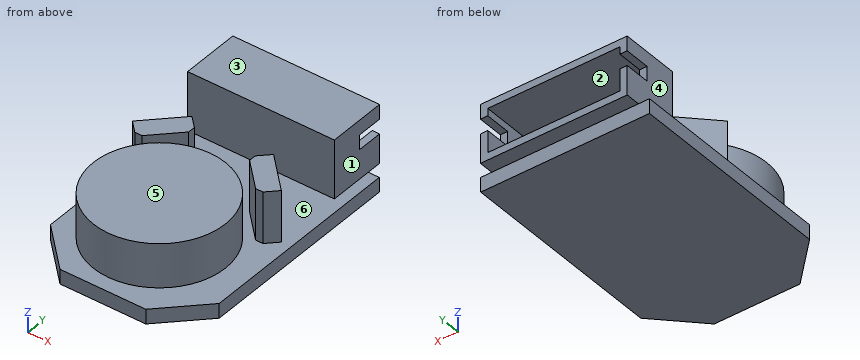
from build123d import *

# Parameters (mm, degrees)
SALIENTE_EXTRUIR1_DEPTH = 1
SALIENTE_EXTRUIR2_DEPTH = 3.5
CROQUIS3_R              = 0.25
SALIENTE_EXTRUIR3_DEPTH = 4.5
CROQUIS4_R              = 4.5
SALIENTE_EXTRUIR4_DEPTH = 3
CROQUIS5_W              = 10
CROQUIS5_H              = 4
SALIENTE_EXTRUIR5_DEPTH = 4
CROQUIS6_W              = 9
CROQUIS6_H              = 3
CORTAR_EXTRUIR1_DEPTH   = 3.5
CROQUIS7_W              = 1
CROQUIS7_H              = 2
CORTAR_EXTRUIR2_DEPTH   = 16.192514604


with BuildPart() as part:
    # Croquis1 → Saliente-Extruir1 (new body)
    with BuildSketch(Plane.XY):
        Polygon((-5.75, -5.671572875), (-2.921572875, -8.5), (2.921572875, -8.5), (5.75, -5.671572875), (5.75, 8.5), (-5.75, 8.5), align=None)
    extrude(amount=SALIENTE_EXTRUIR1_DEPTH)

    # Croquis2 → Saliente-Extruir2 (add)
    with BuildSketch(Plane.XY.offset(1)):
        Polygon((-2.780902327, 3), (-5.073795546, 0.707106781), (-4.366688764, 0), (-3.866688764, 0), (-2.073795546, 1.792893219), (-2.073795546, 2.292893219), align=None)
        Polygon((2.073795546, 1.792893219), (2.073795546, 2.292893219), (2.780902327, 3), (5.073795546, 0.707106781), (4.366688764, 0), (3.866688764, 0), align=None)
    extrude(amount=SALIENTE_EXTRUIR2_DEPTH)

    # Croquis3 → Saliente-Extruir3 (add)
    with BuildSketch(Plane.XY):
        with Locations(Location((0, -3.5, 0), (0, 0, 180))):
            Circle(CROQUIS3_R)
    extrude(amount=SALIENTE_EXTRUIR3_DEPTH)

    # Croquis4 → Saliente-Extruir4 (add)
    with BuildSketch(Plane.XY.offset(4.5)):
        with Locations((0, -3.5)):
            Circle(CROQUIS4_R)
    extrude(amount=-SALIENTE_EXTRUIR4_DEPTH)

    # Croquis5 → Saliente-Extruir5 (add)
    with BuildSketch(Plane.XY.offset(1)):
        with Locations((0, 7.5)):
            Rectangle(CROQUIS5_W, CROQUIS5_H)
    extrude(amount=SALIENTE_EXTRUIR5_DEPTH)

    # Croquis6 → Cortar-Extruir1 (cut)
    with BuildSketch(Plane(origin=(0, 9.5, 0), x_dir=(1, 0, 0), z_dir=(0, 1, 0))):
        with Locations((0, -3)):
            Rectangle(CROQUIS6_W, CROQUIS6_H)
    extrude(amount=-CORTAR_EXTRUIR1_DEPTH, mode=Mode.SUBTRACT)

    # Croquis7 → Cortar-Extruir2 (cut, through all)
    with BuildSketch(Plane(origin=(5, 0, 0), x_dir=(0, 0, -1), z_dir=(1, 0, 0))):
        with Locations((-3.5, 8.741122999)):
            Rectangle(CROQUIS7_W, CROQUIS7_H)
    extrude(amount=-CORTAR_EXTRUIR2_DEPTH, mode=Mode.SUBTRACT)


solid = part.part
Geometry check sheet. Reference: the model listing, model coordinates, mm. Face numbers are marked on the shaded views. A direction names the side the tool comes from. Round coordinates to 2 decimals unless told otherwise and drop trailing zeros. Write each loop counter-clockwise with the first axis right and the second up, starting at its lowest first coordinate (ties: lowest second). Pieces come first, ordered by that corner, then holes. Notation, with made-up numbers: (-40, 6) - (6, 6) arc R18 ccw to (6, 33) - close; hole circle Ø11 at (-8.5, 59). An arc over 180 degrees is marked (long way). One line per item, written item: value.
1. Scan lines: L1, parallel to Y at x = -2.75, z = 3.2; L2, parallel to Z at x = 0, y = 6.75; L3, parallel to Y at x = -3.75, z = 3.5. Record each from-to range of solid material in increasing order.
The answers:
L1: y = -7.06 to 0.06, 1.12 to 2.97, 5.5 to 6
L2: z = 0 to 1.5, 4.5 to 5
L3: y = -5.99 to -1.01, 0.12 to 2.03, 5.5 to 6
2. Mould release check, pull along X, two halves, no side actions. Record for the marked faces 1, 2 and 3: released by +X, released by -X, zero draft, split by the parting line, or undercut.
The answers:
face 1: released by +X
face 2: undercut
face 3: zero draft
3. Cross-section at D-D on z = 0.8. Record the boundary of the cut face in (x, y).
The answers:
outline: (-5.75, -5.67) - (-2.92, -8.5) - (2.92, -8.5) - (5.75, -5.67) - (5.75, 8.5) - (-5.75, 8.5) - close
4. Cross-section at C-C on y = -3.5. Record the boundary of the cut face in (x, z).
The answers:
outline: (-5.75, 0) - (5.75, 0) - (5.75, 1) - (0.25, 1) - (0.25, 1.5) - (4.5, 1.5) - (4.5, 4.5) - (-4.5, 4.5) - (-4.5, 1.5) - (-0.25, 1.5) - (-0.25, 1) - (-5.75, 1) - close
5. Cross-section at A-A on z = 3.3. Record the boundary of the cut face in (x, y).
The answers:
outline: (-5.07, 0.71) - (-4.37, 0) - (-3.87, 0) - (-2.07, 1.79) - (-2.07, 2.29) - (-2.78, 3) - close; (-5, 5.5) - (5, 5.5) - (5, 7.74) - (4.5, 7.74) - (4.5, 6) - (-4.5, 6) - (-4.5, 7.74) - (-5, 7.74) - close; circle Ø9 at (0, -3.5); (2.07, 1.79) - (3.87, 0) - (4.37, 0) - (5.07, 0.71) - (2.78, 3) - (2.07, 2.29) - close
6. Set-up check for the marked faces 4, 5 and 6: record each of +Z, -Z, +X, -X, +Y, -Y from which the full face is reachable in a straight line by a thin tool's end or side.
The answers:
face 4: +Z, -X, +Y
face 5: +Z, +X, -X, -Y
face 6: none
7. Cross-section at B-B on x = 0. Record the boundary of the cut face in (y, z).
The answers:
outline: (-8.5, 0) - (8.5, 0) - (8.5, 1) - (9.5, 1) - (9.5, 1.5) - (6, 1.5) - (6, 4.5) - (9.5, 4.5) - (9.5, 5) - (5.5, 5) - (5.5, 1) - (-3.25, 1) - (-3.25, 1.5) - (1, 1.5) - (1, 4.5) - (-8, 4.5) - (-8, 1.5) - (-3.75, 1.5) - (-3.75, 1) - (-8.5, 1) - close
8. Depth check by flat-ended pin: pin 1 Ø3.5 at (x, y) = (3.5, 1) entering from +Z; pin 2 Ø1.5 at (y, z) = (8, 3) entering from +X; pin 3 Ø0.6 at (x, z) = (-4.5, 3.5) entering from +Y. Enter the tip coordinate at first touch or a pass-through.
The answers:
pin 1: stops at z = 4.5
pin 2: stops at x = 5
pin 3: stops at y = 7.74
